```python
from build123d import *

# Parameters (mm, degrees)
F1_DEPTH  = 25.4
F3_DEPTH  = 101.6
F5_DEPTH  = 101.6
F7_DEPTH  = 101.6
F9_DEPTH  = 127
F11_DEPTH = 101.6
F13_DEPTH = 101.6


with BuildPart() as f1:
    # F0 (on Front) → F1 (new body)
    with BuildSketch(Plane.XZ):
        Polygon((-88.9854516805, 500.1455681991), (0, 0), (381, 0), (292.0145483195, 500.1455681991), align=None)
    extrude(amount=F1_DEPTH)

    # F2 (on face) → F3 (join)
    with BuildSketch(Plane.XZ.offset(25.4)):
        Polygon((-22.5957262885, 127), (0, 0), (381, 0), (358.4042737115, 127), align=None)
    extrude(amount=F3_DEPTH)

    # F4 (on face) → F5 (join)
    with BuildSketch(Plane.XZ.offset(25.4)):
        Polygon((292.0145483195, 500.1455681991), (241.2145483195, 500.1455681991), (241.2145483195, 127), (358.4042737115, 127), align=None)
    extrude(amount=F5_DEPTH)

    # F6 (on face) → F7 (cut)
    with BuildSketch(Plane.XZ.offset(127)):
        Polygon((281.3746764461, 487.4455681991), (253.9145483195, 487.4455681991), (253.9145483195, 139.7), (343.2452565805, 139.7), align=None)
    extrude(amount=-F7_DEPTH, mode=Mode.SUBTRACT)

    # F8 (on face) → F9 (join)
    with BuildSketch(Plane.XZ.offset(127)):
        Polygon((301.3966677113, 447.4130670373), (303.6562403401, 434.7130670373), (381, 434.7130670373), (381, 447.4130670373), align=None)
        Polygon((319.6076049893, 345.0579134663), (321.8671776181, 332.3579134663), (381, 332.3579134663), (381, 345.0579134663), align=None)
        Polygon((343.0322212888, 213.3991107327), (381, 213.3991107327), (381, 226.0991107327), (340.77264866, 226.0991107327), align=None)
    extrude(amount=-F9_DEPTH)

    # F10 (on face) → F11 (join)
    with BuildSketch(Plane.XZ.offset(25.4)):
        Polygon((308.9677331159, 332.3579134663), (306.7081604871, 345.0579134663), (253.9145483195, 345.0579134663), (253.9145483195, 332.3579134663), align=None)
    extrude(amount=F11_DEPTH)

    # F12 (on face) → F13 (join)
    with BuildSketch(Plane.XZ.offset(25.4)):
        Polygon((-9.6962817863, 127), (-76.0860071783, 500.1455681991), (-88.9854516805, 500.1455681991), (-22.5957262885, 127), align=None)
    extrude(amount=F13_DEPTH)


solid = f1.part
```
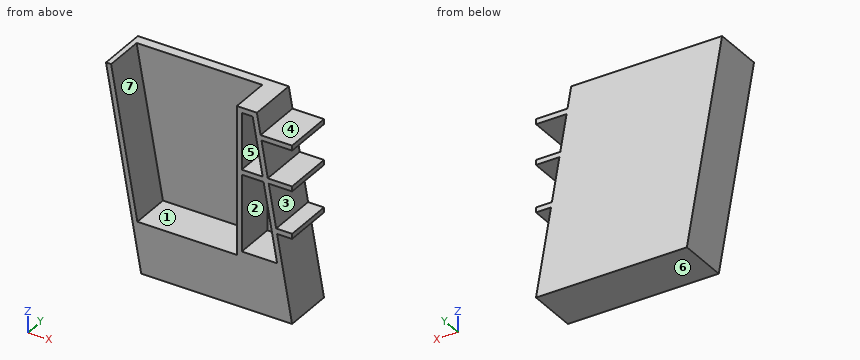
Verification items for the finished model (mm, model axes). Face numbers are marked on the shaded views. A direction names the side the tool comes from. Coordinates: 2 decimals unless noted, no trailing zeros. Order: outer loops, then holes, each group sorted by start corner. A loop starts at its lowest first (then second) coordinate and runs counter-clockwise, first axis right, second up. Notation, with made-up numbers: (48.5, 5.5) - (72.5, 5.5) arc R10 cw to (72.5, 21.5) - close; hole circle Ø10 at (-28.5, 32). An arc over 180 degrees is marked (long way). Return JSON: item names as keys, results as strings.
(1) Section check D-D, the plane x = 101.5. Record the cut outline in (y, z), and give its area (3 significant figures).
Filled sheet:
{"outline": "(-127, 0) - (0, 0) - (0, 500.15) - (-25.4, 500.15) - (-25.4, 127) - (-127, 127) - close", "area": "25,600 mm^2"}
(2) Mould release check, pull along Z, two halves, no side actions. Record for the marked faces 5, 6 and 7: pulls with the +Z half, pulls with the -Z half, needs draft (parallel to the pull), parting line crosses it, or undercut.
Filled sheet:
{"face 5": "undercut", "face 6": "pulls with the -Z half", "face 7": "pulls with the +Z half"}
(3) Access from +Z, -Z, +X, -X, +Y, -Y to the whole of each face (thin tool, end or side, straight path). Record for the marked faces 1, 2, 3 and 4.
Filled sheet:
{"face 1": "+Z, -Y", "face 2": "-Y", "face 3": "+X, +Y, -Y", "face 4": "+Z, +X, +Y, -Y"}
(4) Go/stop test with flat-tipped pins: pin 1 (5 mm diameter, centred on y = -82.5, z = 136.5, fed in from -X); pin 2 (12 mm diameter, centred on y = -74, z = 407.5, fed in from -X); pin 3 (10 mm diameter, centred on x = 20, y = -51.5, fed in from +Z). Record where each tip stops, or that it passes through.
Filled sheet:
{"pin 1": "stops at x = -24.73", "pin 2": "stops at x = -73.57", "pin 3": "stops at z = 127"}
(5) Section check C-C, the plane z = 407. Record the cut outline in (x, y).
Filled sheet:
{"outline": "(-72.41, -127) - (-59.51, -127) - (-59.51, -25.4) - (241.21, -25.4) - (241.21, -127) - (253.91, -127) - (253.91, -25.4) - (295.69, -25.4) - (295.69, -127) - (308.59, -127) - (308.59, 0) - (-72.41, 0) - close"}
(6) Section check B-B, the plane x = 270.5. Record the cut outline in (y, z).
Filled sheet:
{"outline": "(-127, 0) - (0, 0) - (0, 500.15) - (-127, 500.15) - (-127, 487.45) - (-25.4, 487.45) - (-25.4, 345.06) - (-127, 345.06) - (-127, 332.36) - (-25.4, 332.36) - (-25.4, 139.7) - (-127, 139.7) - close"}
(7) Section check A-A, the plane y = -95. Record the cut outline in (x, z).
Filled sheet:
{"outline": "(-88.99, 500.15) - (0, 0) - (381, 0) - (343.03, 213.4) - (381, 213.4) - (381, 226.1) - (340.77, 226.1) - (321.87, 332.36) - (381, 332.36) - (381, 345.06) - (319.61, 345.06) - (303.66, 434.71) - (381, 434.71) - (381, 447.41) - (301.4, 447.41) - (292.01, 500.15) - (241.21, 500.15) - (241.21, 127) - (-9.7, 127) - (-76.09, 500.15) - close; hole (253.91, 139.7) - (343.25, 139.7) - (308.97, 332.36) - (253.91, 332.36) - close; hole (253.91, 345.06) - (306.71, 345.06) - (281.37, 487.45) - (253.91, 487.45) - close"}
(8) Thickness scan on line 1 along Z through (x, y) = (278.5, -93); line 2 along X through (y, z) = (-44, 332); line 3 along X through (y, z) = (-102, 295). Record the ranges inside material, lowest first.
Filled sheet:
{"line 1": "z = 0 to 139.7, 332.36 to 345.06, 487.45 to 500.15", "line 2": "x = -59.07 to -46.17, 241.21 to 253.91, 309.03 to 321.93", "line 3": "x = -52.49 to -39.59, 241.21 to 253.91, 315.61 to 328.51"}
